```python
from build123d import *

# Parameters (mm, degrees)
SKETCH_1_W          = 128.43547374
SKETCH_1_H          = 65.471989544
EXTRUDE_1_DEPTH     = 2
SKETCH_2_W          = 128.43547374
SKETCH_2_H          = 65.471989544
CUT_EXTRUDE_1_DEPTH = 2
SKETCH_3_R          = 2
SKETCH_3_R_2        = 1.9
CUT_EXTRUDE_2_DEPTH = 2


with BuildPart() as part:
    # Sketch 1 → Extrude 1 (new body)
    with BuildSketch(Plane.XY):
        Rectangle(SKETCH_1_W, SKETCH_1_H)
    extrude(amount=EXTRUDE_1_DEPTH)

    # Sketch 2 → Cut-Extrude 1 (cut)
    # profile 1 of 2: a face of its own
    with BuildSketch(Plane(origin=(0, 0, 0), x_dir=(-1, 0, 0), z_dir=(0, 0, -1))):
        Rectangle(SKETCH_2_W, SKETCH_2_H)
        with BuildLine():
            ThreePointArc((-52.204074669, -15.444023491), (-51.848721826, -17.168768362), (-50.267582996, -17.944023491))
            Line((-50.267582996, -17.944023491), (-44.068947588, -17.944023491))
            Line((-44.068947588, -17.944023491), (-33.134584344, -17.944023491))
            ThreePointArc((-33.134584344, -17.944023491), (-19.219474678, -1.055618469), (2.382968092, 2.434792334))
            Line((2.382968092, 2.434792334), (9.266694282, 4.408669056))
            Line((9.266694282, 4.408669056), (9.542331638, 3.44740736))
            Line((9.542331638, 3.44740736), (19.604063858, 6.332562646))
            Line((19.604063858, 6.332562646), (43.186490996, 13.094714813))
            Line((43.186490996, 13.094714813), (42.91085364, 14.055976509))
            Line((42.91085364, 14.055976509), (42.91085364, 18.055976509))
            ThreePointArc((42.91085364, 18.055976509), (42.325067202, 19.470190071), (40.91085364, 20.055976509))
            Line((40.91085364, 20.055976509), (-17.791782842, 20.055976509))
            ThreePointArc((-17.791782842, 20.055976509), (-39.692841918, 6.857039096), (-52.204074669, -15.444023491))
        make_face(mode=Mode.SUBTRACT)
    # profile 2 of 2: a face of its own
    with BuildSketch(Plane(origin=(0, 0, 0), x_dir=(-1, 0, 0), z_dir=(0, 0, -1))):
        with BuildLine():
            ThreePointArc((-12.46838625, 11.103595557), (-11.378536386, 11.760446057), (-10.90548184, 12.941735479))
            ThreePointArc((-10.90548184, 12.941735479), (-11.448173426, 14.429205904), (-12.902216421, 15.055976509))
            Line((-12.902216421, 15.055976509), (-14.562112456, 15.055976509))
            ThreePointArc((-14.562112456, 15.055976509), (-17.300725243, 14.803857713), (-19.947277263, 14.055976509))
            ThreePointArc((-19.947277263, 14.055976509), (-32.344819708, 6.837064556), (-41.840361935, -3.916838284))
            ThreePointArc((-41.840361935, -3.916838284), (-42.583463702, -6.046223655), (-42.315225959, -8.285538463))
            ThreePointArc((-42.315225959, -8.285538463), (-41.764324234, -9.026964046), (-40.939007517, -9.441761496))
            ThreePointArc((-40.939007517, -9.441761496), (-39.67179112, -9.326055361), (-38.730856221, -8.469395089))
            ThreePointArc((-38.730856221, -8.469395089), (-27.694864361, 4.128436562), (-12.46838625, 11.103595557))
        make_face()
    extrude(amount=-CUT_EXTRUDE_1_DEPTH, mode=Mode.SUBTRACT)

    # Sketch 3 → Cut-Extrude 2 (cut)
    with BuildSketch(Plane(origin=(0, 0, 0), x_dir=(-1, 0, 0), z_dir=(0, 0, -1))):
        with Locations((32.208217158, 16.055976509)):
            Circle(SKETCH_3_R)
        with Locations((12.208217158, 16.055976509)):
            Circle(SKETCH_3_R)
        with Locations((-3.791782842, 9.055976509)):
            Circle(SKETCH_3_R_2)
        with Locations((-35.834722782, -9.444023491)):
            Circle(SKETCH_3_R_2)
        with Locations((-22.291782842, 4.098916449)):
            Circle(SKETCH_3_R_2)
    extrude(amount=-CUT_EXTRUDE_2_DEPTH, mode=Mode.SUBTRACT)


solid = part.part
```
Check sheet for the modelled part. Datum: model origin and axes. Units: mm. A direction names the side the tool comes from. Coordinates: 2 decimals unless noted, no trailing zeros. Write each loop counter-clockwise with the first axis right and the second up, starting at its lowest first coordinate (ties: lowest second). Pieces come first, ordered by that corner, then holes. Notation, with made-up numbers: (-27, -23.5) - (-20, -23.5) arc R19 cw to (-20, -2.5) - close; hole circle Ø8 at (13, -33.75). An arc over 180 degrees is marked (long way). One line per question, with ' | ' between items.
Item 1: Mould release check, pull along X, two halves, no side actions. Record for faces 1 (the face through (-34.1, 16.7, 1)), 2 (the face through (4, 6, 2)), 3 (the face through (-42.341, 19.455, 0.986)), 4 (the face through (14, 15.056, 1)): pulls with the +X half, pulls with the -X half, needs draft (parallel to the pull), parting line crosses it, or undercut.
Determined:
face 1: undercut | face 2: needs draft | face 3: pulls with the -X half | face 4: undercut
Item 2: Gauge pin test, flat ends, axial feed: P1, Ø0.8, axis at x = 14, z = 1.5, coming from the -Y side; P2, Ø0.6, axis at y = 16, z = 1, coming from the -X side; P3, Ø3, axis at x = -32.21, y = 16.06, coming from the -Z side. Record the tip position at first contact, or that the pin passes through.
Determined:
P1: stops at y = 1.18 | P2: stops at x = -42.91 | P3: passes through
Item 3: Sectioned sample at B-B on y = -3. Record the boundary of the cut face in (x, z).
Determined:
outline: (22.2, 0) - (35.06, 0) - (35.06, 2) - (22.2, 2) - close; (41.25, 0) - (47.13, 0) - (47.13, 2) - (41.25, 2) - close
Item 4: Thickness scan on line 1 (X direction, y = 16.5, z = 0.4); line 2 (X direction, y = -8, z = 0.15); line 3 (Y direction, x = 15.5, z = 0.2). Record the ranges inside material, lowest first. Write a range as [from, to].
Determined:
line 1: x = [-42.91, -34.16], [-30.26, -14.16], [-10.26, 26.7] | line 2: x = [27.52, 34.6], [37.07, 38.47], [42.41, 49.64] | line 3: y = [0.76, 10.3], [15.03, 20.06]
Item 5: Sectioned sample at A-A on x = 16.5. Record the boundary of the cut face in (y, z), plus the area to 3 significant figures.
Determined:
outline: (0.33, 0) - (9.98, 0) - (9.98, 2) - (0.33, 2) - close; (14.93, 0) - (20.06, 0) - (20.06, 2) - (14.93, 2) - close | area: 29.6 mm2
Item 6: Access from +Z, -Z, +X, -X, +Y, -Y to the whole of each face (thin tool, end or side, straight path). Record for faces 5 (the face through (19.49, -1.213, 0.986)), 6 (the face through (27.88, 3.99, 0.99)), 7 (the face through (-42.911, 16, 1)).
Determined:
face 5: +Z, -Z, -Y | face 6: +Z, -Z | face 7: +Z, -Z, -X, +Y
Item 7: Sectioned sample at D-D on x = -17. Record the boundary of the cut face in (y, z).
Determined:
outline: (5.59, 0) - (20.06, 0) - (20.06, 2) - (5.59, 2) - close
Item 8: Sectioned sample at C-C on z = 0.75. Record the boundary of the cut face in (x, y), plus the area to 3 significant figures.
Determined:
outline: (-43.19, 13.09) - (-9.54, 3.45) - (-9.27, 4.41) - (-2.38, 2.43) arc R31 cw to (33.13, -17.94) - (50.27, -17.94) arc R2 ccw to (52.2, -15.44) arc R50 ccw to (17.79, 20.06) - (-40.91, 20.06) arc R2 ccw to (-42.91, 18.06) - (-42.91, 14.06) - close; hole circle Ø4 at (-32.21, 16.06); hole circle Ø4 at (-12.21, 16.06); hole circle Ø3.8 at (3.79, 9.06); hole (12.47, 11.1) arc R40 cw to (38.73, -8.47) arc R2 ccw to (42.32, -8.29) arc R5 ccw to (41.84, -3.92) arc R45 ccw to (19.95, 14.06) arc R15 ccw to (14.56, 15.06) - (12.9, 15.06) arc R2 ccw to start; hole circle Ø3.8 at (22.29, 4.1); hole circle Ø3.8 at (35.83, -9.44) | area: 1,370 mm2
